Geometry check sheet. Reference: the model listing, model coordinates, mm. A direction names the side the tool comes from. Coordinates: 2 decimals unless noted, no trailing zeros. Order: outer loops, then holes, each group sorted by start corner. A loop starts at its lowest first (then second) coordinate and runs counter-clockwise, first axis right, second up. Notation, with made-up numbers: (-4, 88.5) - (46, 88.5) arc R29 ccw to (46, 124.5) - close; hole circle Ø3 at (29, 80.5). An arc over 180 degrees is marked (long way). Use CSV: the item, a comma, the result in double quotes. Start each with the question number.
1) Tool access check on faces 1 (the flat face through (0, -17, 3)), 2 (the flat face through (51.614, -10.904, 3.76)), 3 (the cylindrical face through (-59.513, -1.943, 3.739)). Record the directions out of +Z, -Z, +X, -X, +Y, -Y that give a thin tool (end or side, any length) a straight path to the whole face; none if there is none.
2) Sectioned sample at B-B, the plane x = -30.5. Record the cut outline in (y, z).
3) Sectioned sample at A-A, the plane z = 1.9. Record the cut outline in (x, y), and give its area (3 significant figures).
4) Thickness scan on probe 1 along Y at (x, z) = (67.5, 4.7); probe 2 along X at (y, z) = (5.75, 0.9); probe 3 along Y at (x, z) = (7, 2.15). Record the ranges inside material, lowest first. Write a range as [from, to].
5) Depth check by flat-ended pin: P1, Ø5, axis at x = -67.5, y = 0, coming from the +Z side; P2, Ø3, axis at y = -16.5, z = 1, coming from the +X side; P3, Ø1.7, axis at x = 4.5, z = 4, coming from the +Y side; P4, Ø1.5, axis at y = -15, z = 3, coming from the +X side. Enter the tip coordinate at first touch or a pass-through.
6) Draft check along Y on faces 4 (the cylindrical face through (51.65, -10.55, 5.2)), 5 (the flat face through (51.016, -4.036, 0.246)), 6 (the cylindrical face through (-65.592, 0.601, 4.268)). Enter one of: released by +Y, released by -Y, zero draft, split by the parting line, or undercut.
from build123d import *

# Parameters (mm, degrees)
EXTRUDE_1_DEPTH       = 2.500000000014097
EXTRUDE_2_DEPTH       = 2.9999999999999996
HOLE_WIZARD_4_0_4_1_D = 4
FILLET_1_R            = 10
FILLET_2_R            = 15.000000000000004
CHAMFER_1_SIZE        = 0.4999999999999998
FILLET_4_R            = 1
EXTRUDE_START         = -3
SKETCH_5_R            = 1.999999999999988
EXTRUDE_3_DEPTH       = 3


with BuildPart() as part:
    # 草图1 → 凸台-拉伸1 (new body)
    with BuildSketch(Plane.XY.offset(5.5)):
        with BuildLine():
            Line((-62.772774424948345, -4.461315765845048), (-41.9211616751135, -16.50000000000001))
            Line((-41.9211616751135, -16.50000000000001), (41.92116167511347, -16.5))
            Line((41.92116167511347, -16.5), (62.77277442494833, -4.461315765845017))
            ThreePointArc((62.77277442494833, -4.461315765845017), (73.12916512459886, 3.249999999999975), (61.27277442494834, -1.863239554491695))
            Line((61.27277442494834, -1.863239554491695), (41.117314097820056, -13.50000000000001))
            Line((41.117314097820056, -13.50000000000001), (-41.117314097820156, -13.500000000000009))
            Line((-41.117314097820156, -13.500000000000009), (-61.272774424948345, -1.863239554491729))
            ThreePointArc((-61.272774424948345, -1.863239554491729), (-73.12916512459884, 3.2500000000000075), (-62.772774424948345, -4.461315765845048))
        make_face()
    extrude(amount=-EXTRUDE_1_DEPTH)

    # 草图2 → 凸台-拉伸2 (add)
    with BuildSketch(Plane(origin=(0, 0, 2.9999999999859024), x_dir=(-1, 0, 0), z_dir=(0, 0, -1))):
        with BuildLine():
            Line((66.40312635751548, -6.406782984651714), (42.858983848622465, -20))
            Line((42.858983848622465, -20), (-42.85898384862241, -19.999999999999996))
            Line((-42.85898384862241, -19.999999999999996), (-66.40312635751543, -6.406782984651706))
            ThreePointArc((-66.40312635751543, -6.406782984651706), (-73.12916512459887, 3.24999999999996), (-61.40312635751548, 2.253471053192728))
            Line((-61.40312635751548, 2.253471053192728), (-40.17949192431118, -9.999999999999998))
            Line((-40.17949192431118, -9.999999999999998), (40.17949192431122, -10.000000000000009))
            Line((40.17949192431122, -10.000000000000009), (61.40312635751546, 2.2534710531926625))
            ThreePointArc((61.40312635751546, 2.2534710531926625), (73.12916512459884, 3.250000000000009), (66.40312635751548, -6.406782984651714))
        make_face()
    extrude(amount=EXTRUDE_2_DEPTH)

    # Ø4.0 (4) 直径孔1 (through all)
    with Locations(Plane(origin=(0, 0, 0), x_dir=(-1, 0, 0), z_dir=(0, 0, -1))):
        with Locations((67.5, 0), (-67.5, 0)):
            Hole(HOLE_WIZARD_4_0_4_1_D / 2)

    # 圆角1
    fillet_1_edges = [part.edges().sort_by_distance(p)[0] for p in [
        (-61.27277442494835, -1.8632395544917282, 4.249999999992951),
        (-41.117314097820156, -13.500000000000009, 4.249999999992951),
        (41.117314097820056, -13.50000000000001, 4.249999999992951),
        (61.27277442494834, -1.863239554491694, 4.249999999992951),
        (62.77277442494834, -4.461315765845014, 4.249999999992951),
        (-62.772774424948345, -4.461315765845047, 4.249999999992951),
        (-66.40312635751548, -6.406782984651716, 1.4999999999859026),
        (-61.40312635751547, 2.2534710531926603, 1.4999999999859026),
        (-40.17949192431122, -10.000000000000009, 1.4999999999859026),
        (40.17949192431118, -9.999999999999998, 1.4999999999859026),
        (61.403126357515475, 2.2534710531927282, 1.4999999999859026),
        (66.40312635751543, -6.406782984651702, 1.4999999999859026),
    ]]
    fillet(fillet_1_edges, radius=FILLET_1_R)

    # 圆角2
    fillet_2_edges = [part.edges().sort_by_distance(p)[0] for p in [
        (41.92116167511347, -16.5, 4.249999999992951),
        (-41.9211616751135, -16.50000000000001, 4.249999999992951),
        (42.85898384862241, -19.999999999999996, 1.4999999999859026),
        (-42.858983848622465, -20, 1.4999999999859026),
    ]]
    fillet(fillet_2_edges, radius=FILLET_2_R)

    # 倒角1
    chamfer_1_edges = [part.edges().sort_by_distance(p)[0] for p in [
        (-55.193402756130126, -12.878719923452845, -1.409717e-11),
        (-1.421e-14, -19.999999999999996, -1.409717e-11),
        (42.722031638693394, -19.488887394336025, -1.409717e-11),
        (-42.72203163869342, -19.48888739433603, -1.409717e-11),
        (50.77352977505234, -3.883529395069502, -1.409717e-11),
        (-2.132e-14, -10.000000000000004, -1.409717e-11),
        (-50.77352977505235, -3.8835293950695364, -1.409717e-11),
        (-73.12916512459887, 3.2499999999999756, -1.409717e-11),
        (55.193402756130126, -12.878719923452813, -1.409717e-11),
        (73.12916512459886, 3.2499999999999876, -1.409717e-11),
        (40.088190451025156, -9.659258262890683, -1.409717e-11),
        (-60.778474019386664, 2.158311745061262, -1.409717e-11),
        (66.00838981020269, -6.900168123938897, -1.409717e-11),
        (-40.08819045102521, -9.65925826289069, -1.409717e-11),
        (60.778474019386664, 2.1583117450613107, -1.409717e-11),
        (-66.00838981020267, -6.900168123938933, -1.409717e-11),
    ]]
    chamfer(chamfer_1_edges, length=CHAMFER_1_SIZE)

    # 圆角4
    fillet_4_edges = [part.edges().sort_by_distance(p)[0] for p in [
        (-1.421e-14, -16.500000000000004, 5.5),
        (51.70248651134352, -10.85274947277141, 5.5),
        (-41.784209465184475, -15.988887394336034, 5.5),
        (41.78420946518445, -15.988887394336027, 5.5),
        (-73.12916512459887, 3.2499999999999796, 5.5),
        (73.12916512459886, 3.250000000000003, 5.5),
        (49.970435703774626, -8.388647857633657, 5.5),
        (-4.974e-14, -13.50000000000001, 5.5),
        (-49.970435703774676, -8.388647857633675, 5.5),
        (-51.70248651134354, -10.852749472771439, 5.5),
        (59.47971041107501, -1.9877806313493807, 5.5),
        (-41.02601262453415, -13.159258262890692, 5.5),
        (-59.479710411075004, -1.9877806313494268, 5.5),
        (-61.76838668163823, -5.951884214042208, 5.5),
        (61.76838668163825, -5.951884214042176, 5.5),
        (41.02601262453404, -13.159258262890695, 5.5),
    ]]
    fillet(fillet_4_edges, radius=FILLET_4_R)

    # 草图5 → 凸台-拉伸3 (add)
    with BuildSketch(Plane(origin=(0, 0, 0), x_dir=(-1, 0, 0), z_dir=(0, 0, -1)).offset(EXTRUDE_START)):
        with Locations((67.5, 0)):
            Circle(SKETCH_5_R)
        with Locations((-67.5, 0)):
            Circle(SKETCH_5_R)
    extrude(amount=EXTRUDE_3_DEPTH)


solid = part.part
Evaluation:
1,face 1,"+Z, -Y"
1,face 2,"+Z, +X, -Y"
1,face 3,"+Z, +Y"
2,outline,"(-20, 0.5) - (-19.5, 0) - (-10.5, 0) - (-10, 0.5) - (-10, 3) - (-13.5, 3) - (-13.5, 4.5) arc R1 ccw to (-14.5, 5.5) - (-15.5, 5.5) arc R1 ccw to (-16.5, 4.5) - (-16.5, 3) - (-20, 3) - close"
3,outline,"(-68.11, -6.47) arc R10 cw to (-64.05, -7.77) - (-46.34, -17.99) arc R15 ccw to (-38.84, -20) - (38.84, -20) arc R15 ccw to (46.34, -17.99) - (64.05, -7.77) arc R10 cw to (68.11, -6.47) arc R6.5 ccw (long way) to (62.2, 3.76) arc R10 cw to (59.05, 0.89) - (42.5, -8.66) arc R10 cw to (37.5, -10) - (-37.5, -10) arc R10 cw to (-42.5, -8.66) - (-59.05, 0.89) arc R10 cw to (-62.2, 3.76) arc R6.5 ccw (long way) to start"
3,area,"1,580 mm²"
4,probe 1,"[-6.48, -2], [2, 6.48]"
4,probe 2,"[-70.53, -64.47], [64.47, 70.53]"
4,probe 3,"[-20, -10]"
5,P1,"z = 5.5"
5,P2,"x = 51.52"
5,P3,"y = -13.5"
5,P4,"x = 52.82"
6,face 4,"released by -Y"
6,face 5,"released by +Y"
6,face 6,"undercut"
